Drawing for the job (mm, zero at the part's lowest x, y, z). A direction names the side the tool comes from. Round coordinates to 2 decimals unless told otherwise and drop trailing zeros. Loops run counter-clockwise (first coordinate to the right, second up) from the corner with the lowest first, then second, coordinate; pieces in that order, holes last. Notation, with made-up numbers: (6, -30.75) - (44, -30.75) arc R22 cw to (44, -11.75) - close; hole circle Ø4 at (58.5, -32). An arc over 180 degrees is marked (long way). Put each result on its own line as item: value.
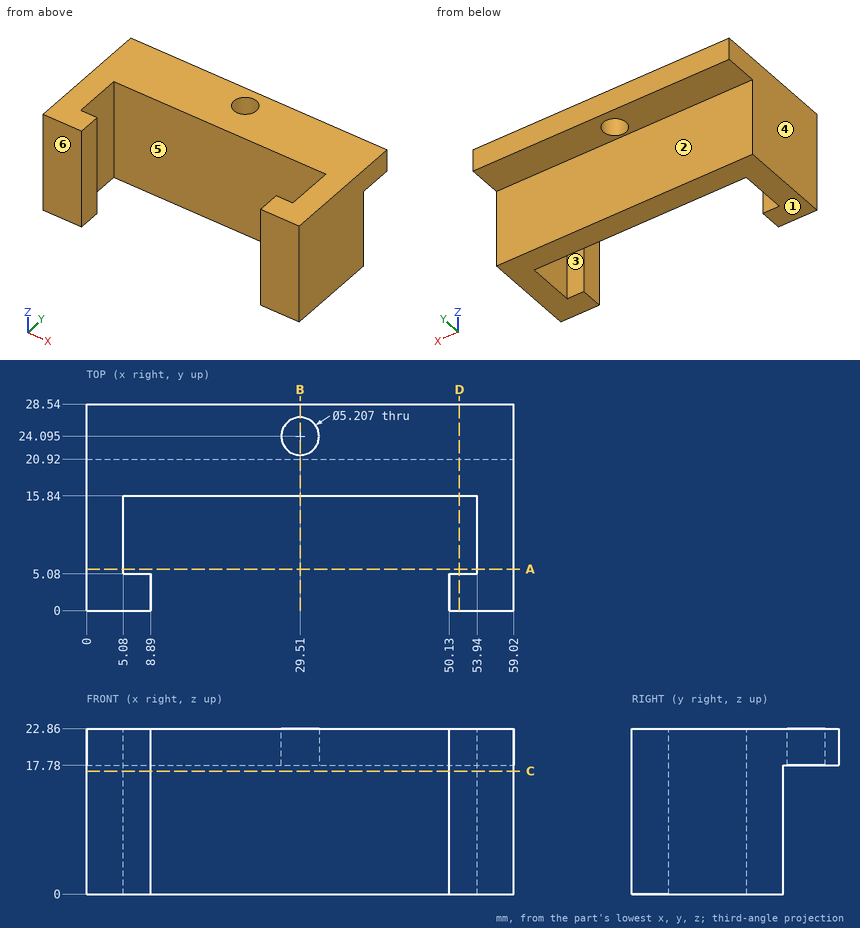
1. Band-saw the part on A-A (y = 5.75). List the corners of the cut face in (x, z).
A:
outline: (0, 0) - (5.08, 0) - (5.08, 22.86) - (0, 22.86) - close; (53.94, 0) - (59.02, 0) - (59.02, 22.86) - (53.94, 22.86) - close
2. Band-saw the part on C-C (z = 17). List the corners of the cut face in (x, y).
A:
outline: (0, 0) - (8.89, 0) - (8.89, 5.08) - (5.08, 5.08) - (5.08, 15.84) - (53.94, 15.84) - (53.94, 5.08) - (50.13, 5.08) - (50.13, 0) - (59.02, 0) - (59.02, 20.92) - (0, 20.92) - close
3. Pin check, flat tips, straight feed: P1, Ø4, axis at x = 52, z = 15, coming from the +Y side; P2, Ø4, axis at x = 37.5, y = 24.5, coming from the -Z side; P3, Ø5, axis at x = 30.5, z = 19.5, coming from the -Y side. Stop position of each tip, or through.
A:
P1: stops at y = 20.92
P2: stops at z = 17.78
P3: stops at y = 15.84
4. Two-plate mould, pull along X, no slides. Class the marked faces 4, 5 and 6: pulls with the +X half, pulls with the -X half, needs draft (parallel to the pull), parting line crosses it, or undercut.
A:
face 4: pulls with the -X half
face 5: undercut
face 6: needs draft
5. Band-saw the part on B-B (x = 29.51). List the corners of the cut face in (y, z), plus the area to 3 significant figures.
A:
outline: (15.84, 0) - (20.92, 0) - (20.92, 17.78) - (21.49, 17.78) - (21.49, 22.86) - (15.84, 22.86) - close; (26.7, 17.78) - (28.54, 17.78) - (28.54, 22.86) - (26.7, 22.86) - close
area: 128 mm²
6. Probe line 1 along X through (y, z) = (9.5, 16.25); line 2 along X through (y, z) = (4.5, 3.75); line 3 along Y through (x, z) = (29.51, 19.8). List the from-to ranges inside material, lowest first. Write a range as [from, to].
A:
line 1: x = [0, 5.08], [53.94, 59.02]
line 2: x = [0, 8.89], [50.13, 59.02]
line 3: y = [15.84, 21.49], [26.7, 28.54]
7. Tool access for the marked faces 1, 2 and 3: list every direction of +Z, -Z, +X, -X, +Y, -Y with a clear straight run to the whole face (end or side of a thin tool).
A:
face 1: -Z, +X, -X, +Y, -Y
face 2: -Z, +X, -X, +Y
face 3: +Z, -Z
8. Band-saw the part on D-D (x = 51.5). List the corners of the cut face in (y, z).
A:
outline: (0, 0) - (5.08, 0) - (5.08, 22.86) - (0, 22.86) - close; (15.84, 0) - (20.92, 0) - (20.92, 17.78) - (28.54, 17.78) - (28.54, 22.86) - (15.84, 22.86) - close
